Verification items for the finished model (mm, model axes). A direction names the side the tool comes from. Coordinates: 2 decimals unless noted, no trailing zeros. Write each loop counter-clockwise with the first axis right and the second up, starting at its lowest first coordinate (ties: lowest second). Pieces come first, ordered by that corner, then holes. Notation, with made-up numbers: (22, 33) - (67, 33) arc R27 ccw to (67, 57) - close; hole circle Ø4 at (58.5, 29). An arc over 180 degrees is marked (long way). Use one line per item in the form item = value. Start each with the question number.
(1) Tool access check on faces 1 (the cylindrical face through (-15.24, -6.32, -11.19)), 2 (the flat face through (0, 7, 43.5)), 3 (the flat face through (1, 10, 28)). Record the directions out of +Z, -Z, +X, -X, +Y, -Y that give a thin tool (end or side, any length) a straight path to the whole face; none if there is none.
(2) Material ranges on line 1 (Z direction, x = 2, y = -5); line 2 (Z direction, x = 11, y = -14); line 3 (Y direction, x = 0.5, z = 23), recorded low to high. Write a range as [from, to].
(3) Gauge pin test, flat ends, axial feed: pin 1 Ø12 at (x, y) = (4.5, 0) entering from +Z; pin 2 Ø3 at (y, z) = (-1, -4.5) entering from +X; pin 3 Ø6 at (x, z) = (-3.5, 1.5) entering from +Y; pin 4 Ø12 at (x, z) = (6.5, -13.5) entering from +Y. Record the tip position at first contact, or that the pin passes through.
(4) Sectioned sample at A-A (x = 0). Record the cut outline in (y, z), and give its area (3 significant figures).
(5) Sectioned sample at D-D (x = 10). Record the cut outline in (y, z).
(6) Sectioned sample at C-C (z = 35.5). Record the cut outline in (x, y), and give its area (3 significant figures).
(7) Sectioned sample at B-B (y = 0). Record the cut outline in (x, z), and give its area (3 significant figures).
from build123d import *

# Parameters (mm, degrees)
SKETCH1_R           = 18.5
BOSS_EXTRUDE1_DEPTH = 22
SKETCH2_R           = 6
BOSS_EXTRUDE2_DEPTH = 6
SKETCH3_R           = 3
BOSS_EXTRUDE3_DEPTH = 15.5
SKETCH4_R           = 16.5
BOSS_EXTRUDE4_DEPTH = 22.7


with BuildPart() as part:
    # Sketch1 → Boss-Extrude1 (new body)
    with BuildSketch(Plane.XY):
        Circle(SKETCH1_R)
    extrude(amount=BOSS_EXTRUDE1_DEPTH)

    # Sketch2 → Boss-Extrude2 (add)
    with BuildSketch(Plane.XY.offset(22)):
        with Locations((0, 7)):
            Circle(SKETCH2_R)
    extrude(amount=BOSS_EXTRUDE2_DEPTH)

    # Sketch3 → Boss-Extrude3 (add)
    with BuildSketch(Plane.XY.offset(28)):
        with Locations((0, 7)):
            Circle(SKETCH3_R)
    extrude(amount=BOSS_EXTRUDE3_DEPTH)

    # Sketch4 → Boss-Extrude4 (add)
    with BuildSketch(Plane(origin=(0, 0, 0), x_dir=(-1, 0, 0), z_dir=(0, 0, -1))):
        Circle(SKETCH4_R)
    extrude(amount=BOSS_EXTRUDE4_DEPTH)


solid = part.part
Answers below:
q1.face_1 = -Z
q1.face_2 = +Z, +X, -X, +Y, -Y
q1.face_3 = +Z
q2.line_1 = [-22.7, 22]
q2.line_2 = [0, 22]
q2.line_3 = [1.02, 12.98]
q3.pin_1 = 43.5
q3.pin_2 = 16.5
q3.pin_3 = 18.49
q3.pin_4 = 16.49
q4.outline = (-18.5, 0) - (-16.5, 0) - (-16.5, -22.7) - (16.5, -22.7) - (16.5, 0) - (18.5, 0) - (18.5, 22) - (13, 22) - (13, 28) - (10, 28) - (10, 43.5) - (4, 43.5) - (4, 28) - (1, 28) - (1, 22) - (-18.5, 22) - close
q4.area = 1,730 mm2
q5.outline = (-15.56, 0) - (-13.12, 0) - (-13.12, -22.7) - (13.12, -22.7) - (13.12, 0) - (15.56, 0) - (15.56, 22) - (-15.56, 22) - close
q6.outline = circle Ø6 at (0, 7)
q6.area = 28.3 mm2
q7.outline = (-18.5, 0) - (-16.5, 0) - (-16.5, -22.7) - (16.5, -22.7) - (16.5, 0) - (18.5, 0) - (18.5, 22) - (-18.5, 22) - close
q7.area = 1,560 mm2
